The model under review builds one solid part; all positions refer to its coordinate system, in mm. Coordinates: 2 decimals unless noted, no trailing zeros. Write each loop counter-clockwise with the first axis right and the second up, starting at its lowest first coordinate (ties: lowest second). Pieces come first, ordered by that corner, then holes.
Solid Edge part; units mm, degrees
sketch "Sketch1" plane through (0, 0, 0) normal (0, 0, 1) x (1, 0, 0)
  line L0 (24.8709, 23.0576) -> (29.1209, 30.4188)
  line L1 (29.1209, 30.4188) -> (37.6209, 30.4188)
  line L2 (37.6209, 30.4188) -> (41.8709, 23.0576)
  line L3 (41.8709, 23.0576) -> (37.3297, 16.2008)
  line L4 (37.3297, 16.2008) -> (29.1209, 15.6964)
  line L5 (29.1209, 15.6964) -> (24.8709, 23.0576)
extrude "Protrusion1" add sketch "Sketch1" against normal blind 6
sketch "Sketch2" plane through (33.3709, 23.0576, -6) normal (0, 0, -1) x (-0.5, 0.866, 0)
  circle A0 centre (0, 0) radius 5
extrude "ExtrudedCutout_2" cut sketch "Sketch2" against normal blind 6
Item 1: Mouldability with a two-part tool opening along Z and no side actions: class faces 1 (the face through (31.6, 28.1, -6)), 2 (the face through (31.6, 28.1, 0)), 3 (the face through (26.97, 26.69, -2.96)) as pulls with the +Z half, pulls with the -Z half, needs draft (parallel to the pull), parting line crosses it, or undercut.
Solved:
face 1: pulls with the -Z half
face 2: pulls with the +Z half
face 3: needs draft
Item 2: Take a section at B-B, the plane x = 30. Write out the cut boundary in (y, z), plus the area to 3 significant figures.
Solved:
outline: (15.75, -6) - (19.36, -6) - (19.36, 0) - (15.75, 0) - close; (26.75, -6) - (30.42, -6) - (30.42, 0) - (26.75, 0) - close
area: 43.7 mm2
Item 3: Take a section at C-C, the plane z = -2.5. Write out the cut boundary in (x, y), plus the area to 3 significant figures.
Solved:
outline: (24.87, 23.06) - (29.12, 15.7) - (37.33, 16.2) - (41.87, 23.06) - (37.62, 30.42) - (29.12, 30.42) - close; hole circle Ø10 at (33.37, 23.06)
area: 105 mm2
Item 4: Take a section at A-A, the plane y = 23.5. Write out the cut boundary in (x, z), plus the area to 3 significant figures.
Solved:
outline: (25.13, -6) - (28.39, -6) - (28.39, 0) - (25.13, 0) - close; (38.35, -6) - (41.62, -6) - (41.62, 0) - (38.35, 0) - close
area: 39.2 mm2
Item 5: Take a section at D-D, the plane y = 29.25. Write out the cut boundary in (x, z), plus the area to 3 significant figures.
Solved:
outline: (28.45, -6) - (38.3, -6) - (38.3, 0) - (28.45, 0) - close
area: 59.1 mm2
Item 6: To check wall thickness, follow line 1 along Y through (x, z) = (36, -3.4); line 2 along Y through (x, z) = (34.5, -4.05); line 3 along X through (y, z) = (27.25, -3.8). State the ranges of each line that lie inside material, in increasing order.
Solved:
line 1: y = 16.12 to 18.8, 27.31 to 30.42
line 2: y = 16.03 to 18.19, 27.93 to 30.42
line 3: x = 27.29 to 30.65, 36.1 to 39.45
Item 7: For pin 1 (2 mm diameter, centred on y = 19, z = -1.5, fed in from +X); pin 2 (4 mm diameter, centred on x = 33, y = 25.5, fed in from -Z), all flat-tipped, find the tip position at first contact; note any pin that passes through.
Solved:
pin 1: stops at x = 39.85
pin 2: passes through
